Geometry check sheet. Reference: the model listing, model coordinates, mm. Face numbers are marked on the shaded views. A direction names the side the tool comes from. Round coordinates to 2 decimals unless told otherwise and drop trailing zeros. Order: outer loops, then holes, each group sorted by start corner. A loop starts at its lowest first (then second) coordinate and runs counter-clockwise, first axis right, second up.
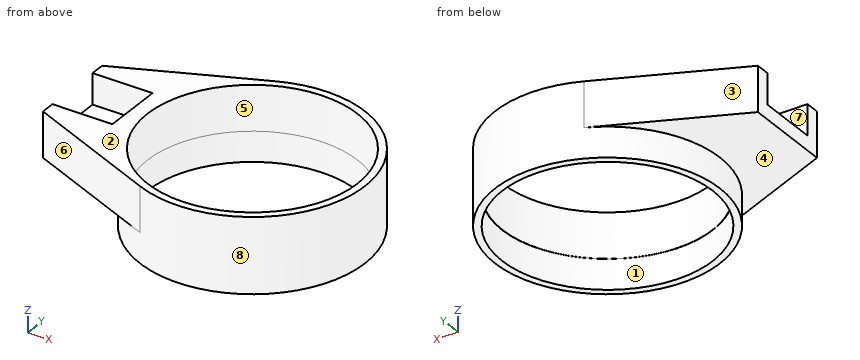
```python
from build123d import *

# Parameters (mm, degrees)
ESQUISSE1_R             = 37.5
ESQUISSE1_R_2           = 35.1
BOSS_EXTRU_1_DEPTH      = 10
ESQUISSE2_R             = 35
BOSS_EXTRU_2_DEPTH      = 15
ESQUISSE6_W             = 10.2
ESQUISSE6_H             = 20.4
ENL_V_MAT_EXTRU_1_DEPTH = 20


with BuildPart() as part:
    # Esquisse1 → Boss.-Extru.1 (new body)
    with BuildSketch(Plane.XY):
        Circle(ESQUISSE1_R)
        Circle(ESQUISSE1_R_2, mode=Mode.SUBTRACT)
    extrude(amount=BOSS_EXTRU_1_DEPTH)

    # Esquisse2 → Boss.-Extru.2 (add)
    with BuildSketch(Plane.XY.offset(10)):
        with BuildLine():
            Line((-60, -15), (-60, 15))
            Line((-60, 15), (-14.826354569, 34.444581725))
            ThreePointArc((-14.826354569, 34.444581725), (37.5, 0), (-14.826354569, -34.444581725))
            Line((-14.826354569, -34.444581725), (-60, -15))
        make_face()
        Circle(ESQUISSE2_R, mode=Mode.SUBTRACT)
    extrude(amount=BOSS_EXTRU_2_DEPTH)

    # Esquisse6 → Enlèv. mat.-Extru.1 (cut)
    with BuildSketch(Plane.ZY.offset(60)):
        with Locations((19.9, 0)):
            Rectangle(ESQUISSE6_W, ESQUISSE6_H)
    extrude(amount=-ENL_V_MAT_EXTRU_1_DEPTH, mode=Mode.SUBTRACT)


solid = part.part
```
(1) Draft check along Y on the marked faces 1, 2 and 3. Enter one of: released by +Y, released by -Y, zero draft, split by the parting line, or undercut.
Returned:
face 1: undercut
face 2: zero draft
face 3: released by +Y
(2) Sectioned sample at C-C, the plane y = 0. Record the cut outline in (x, z).
Returned:
outline: (-60, 10) - (-37.5, 10) - (-37.5, 0) - (-35.1, 0) - (-35.1, 10) - (-35, 10) - (-35, 25) - (-40, 25) - (-40, 14.8) - (-60, 14.8) - close; (35, 10) - (35.1, 10) - (35.1, 0) - (37.5, 0) - (37.5, 25) - (35, 25) - close
(3) Depth check by flat-ended pin: P1, Ø3, axis at y = 18.5, z = 3.5, coming from the -X side; P2, Ø12, axis at x = -8, z = 9.5, coming from the +Y side; P3, Ø11, axis at x = -53.5, z = 17.5, coming from the -Y side. Enter the tip coordinate at first touch or a pass-through.
Returned:
P1: stops at x = -33.43
P2: stops at y = 37.45
P3: stops at y = -20.17
(4) Set-up check for the marked faces 4, 5, 6, 7 and 8: record each of +Z, -Z, +X, -X, +Y, -Y from which the full face is reachable in a straight line by a thin tool's end or side.
Returned:
face 4: -Z, -X
face 5: +Z, -Z
face 6: +Z, -Z, -X, -Y
face 7: +Z, -X
face 8: -Z
(5) Sectioned sample at D-D, the plane y = -26.5. Record the cut outline in (x, z), and give its area (3 significant figures).
Returned:
outline: (-33.28, 10) - (-26.53, 10) - (-26.53, 0) - (-23.02, 0) - (-23.02, 10) - (-22.86, 10) - (-22.86, 25) - (-33.28, 25) - close; (22.86, 10) - (23.02, 10) - (23.02, 0) - (26.53, 0) - (26.53, 25) - (22.86, 25) - close
area: 282 mm2
(6) Sectioned sample at A-A, the plane z = 23.75. Record the cut outline in (x, y).
Returned:
outline: (-60, -15) - (-14.83, -34.44) arc R37.5 ccw (long way) to (-14.83, 34.44) - (-60, 15) - (-60, 10.2) - (-40, 10.2) - (-40, -10.2) - (-60, -10.2) - close; hole circle Ø70 at (0, 0)
(7) Sectioned sample at B-B, the plane x = 0. Record the cut outline in (y, z).
Returned:
outline: (-37.5, 0) - (-35.1, 0) - (-35.1, 10) - (-35, 10) - (-35, 25) - (-37.5, 25) - close; (35, 10) - (35.1, 10) - (35.1, 0) - (37.5, 0) - (37.5, 25) - (35, 25) - close
(8) Material ranges on line 1 (Y direction, x = 0, z = 6); line 2 (Z direction, x = -45, y = 18); line 3 (X direction, y = 2, z = 17.5), recorded low to high.
Returned:
line 1: y = -37.5 to -35.1, 35.1 to 37.5
line 2: z = 10 to 25
line 3: x = -40 to -34.94, 34.94 to 37.45
